For this review, use the dimensioned drawing (mm, ordinates from the lowest corner) and the shaded views. Give positions to 0.01 mm unless a question says otherwise; leave off trailing zeros. Loops run counter-clockwise (first coordinate to the right, second up) from the corner with the lowest first, then second, coordinate; pieces in that order, holes last. Notation, with made-up numbers: (22.25, 70.25) -> (74.25, 70.25) arc R5 ccw to (74.25, 76.25) -> close; hole circle Ø3 at (36, 43). An arc over 180 degrees is marked (long way). Use a Markdown table: item, result. Add a question column.
1. Add section B-B (y = 0.5). State the section outline as (x, z) points.
2. Add section A-A (x = 5). State the section outline as (y, z) points, and give its area (3 significant figures).
3. To check wall thickness, follow line 1 (Z direction, x = 5, y = 2.15); line 2 (X direction, y = 0.85, z = 13); line 3 (Z direction, x = 3, y = 0.5). State the ranges of each line that lie inside material, in increasing order.
4. Add section C-C (z = 8.25). State the section outline as (x, y) points, and give its area (3 significant figures).
5. Add section D-D (x = 9.25). State the section outline as (y, z) points.
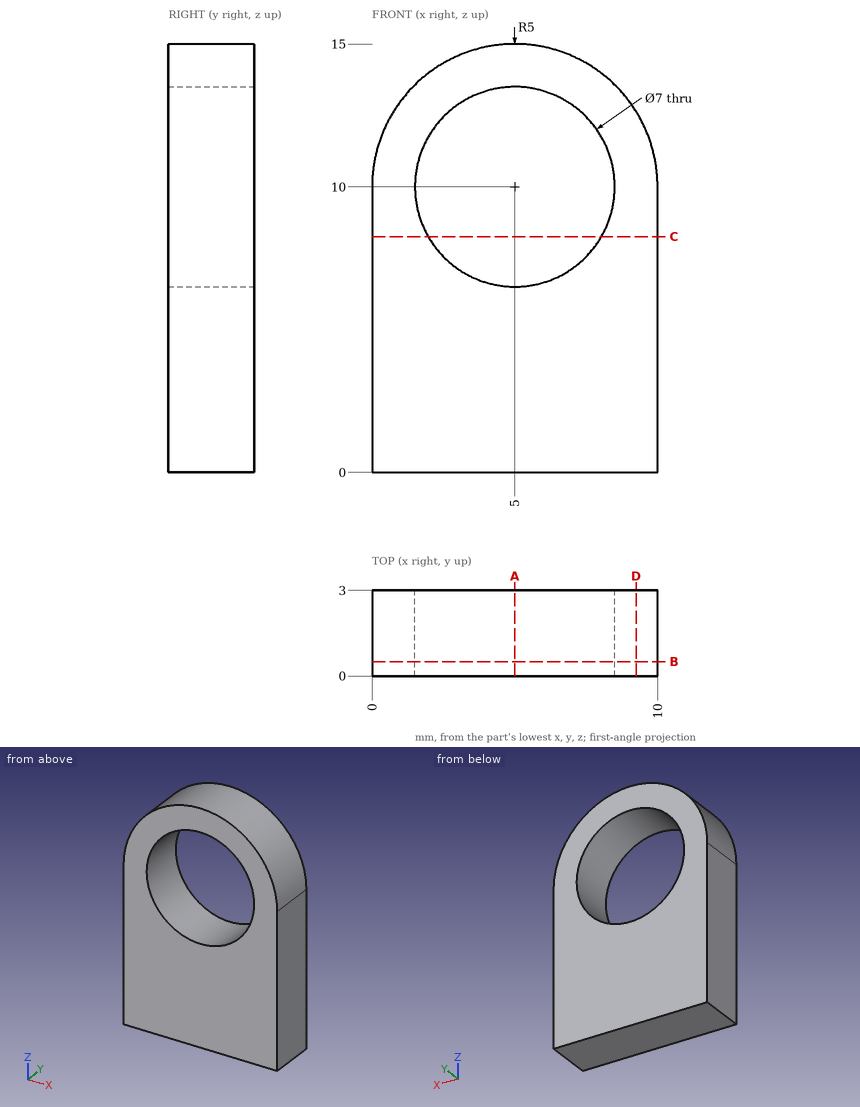
Taken from the geometry:
| question | item | result |
|---|---|---|
| 1 | outline | (0, 0) -> (10, 0) -> (10, 10) arc R5 ccw to (0, 10) -> close; hole circle Ø7 at (5, 10) |
| 2 | outline | (0, 0) -> (3, 0) -> (3, 6.5) -> (0, 6.5) -> close; (0, 13.5) -> (3, 13.5) -> (3, 15) -> (0, 15) -> close |
| 2 | area | 24.0 mm^2 |
| 3 | line 1 | z = 0 to 6.5, 13.5 to 15 |
| 3 | line 2 | x = 1 to 3.2, 6.8 to 9 |
| 3 | line 3 | z = 0 to 7.13, 12.87 to 14.58 |
| 4 | outline | (0, 0) -> (1.97, 0) -> (1.97, 3) -> (0, 3) -> close; (8.03, 0) -> (10, 0) -> (10, 3) -> (8.03, 3) -> close |
| 4 | area | 11.8 mm^2 |
| 5 | outline | (0, 0) -> (3, 0) -> (3, 12.63) -> (0, 12.63) -> close |
